Here's how the part is built. I have some questions about the finished solid (model axes, mm). Round coordinates to 2 decimals unless told otherwise and drop trailing zeros. Order: outer loops, then holes, each group sorted by start corner. A loop starts at its lowest first (then second) coordinate and runs counter-clockwise, first axis right, second up.
```python
from build123d import *

# Parameters (mm, degrees)
SKETCH1_W           = 202
SKETCH1_H           = 152
SKETCH1_R           = 7.5
BOSS_EXTRUDE1_DEPTH = 10
SKETCH2_R           = 25.4
SKETCH2_R_2         = 23.9
BOSS_EXTRUDE2_DEPTH = 1220


with BuildPart() as part:
    # Sketch1 → Boss-Extrude1 (new body)
    with BuildSketch(Plane.XY):
        with Locations((-101, 76)):
            Rectangle(SKETCH1_W, SKETCH1_H)
        with Locations((-185, 141)):
            Circle(SKETCH1_R, mode=Mode.SUBTRACT)
        with Locations((-185, 11)):
            Circle(SKETCH1_R, mode=Mode.SUBTRACT)
        with Locations((-38.177870513, 141)):
            Circle(SKETCH1_R, mode=Mode.SUBTRACT)
        with Locations((-38.177870513, 11)):
            Circle(SKETCH1_R, mode=Mode.SUBTRACT)
    extrude(amount=BOSS_EXTRUDE1_DEPTH)

    # Sketch2 → Boss-Extrude2 (add)
    with BuildSketch(Plane.XY.offset(10)):
        with Locations((-101, 76)):
            Circle(SKETCH2_R)
        with Locations((-101, 76)):
            Circle(SKETCH2_R_2, mode=Mode.SUBTRACT)
    extrude(amount=BOSS_EXTRUDE2_DEPTH)


solid = part.part
```
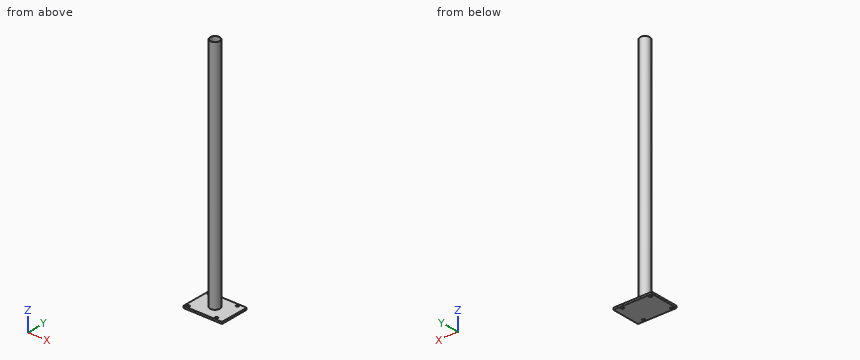
1. If we section it at A-A, the plane y = 76: Write out the boundary of the cut face in (x, z).
Evaluation:
outline: (-202, 0) - (0, 0) - (0, 10) - (-75.6, 10) - (-75.6, 1230) - (-77.1, 1230) - (-77.1, 10) - (-124.9, 10) - (-124.9, 1230) - (-126.4, 1230) - (-126.4, 10) - (-202, 10) - close
2. If we section it at C-C, the plane z = 625: Write out the boundary of the cut face in (x, y).
Evaluation:
outline: circle Ø50.8 at (-101, 76); hole circle Ø47.8 at (-101, 76)
3. I need wall thicknesses on probe 1 along Y at (x, z) = (-185, 6.75); probe 2 along X at (y, z) = (73, 988.5); probe 3 along Y at (x, z) = (-101, 818). Which ranges of each line are inside material? Lowest first, please.
Evaluation:
probe 1: y = 0 to 3.5, 18.5 to 133.5, 148.5 to 152
probe 2: x = -126.22 to -124.71, -77.29 to -75.78
probe 3: y = 50.6 to 52.1, 99.9 to 101.4
4. If we section it at B-B, the plane x = -101: Write out the boundary of the cut face in (y, z).
Evaluation:
outline: (0, 0) - (152, 0) - (152, 10) - (101.4, 10) - (101.4, 1230) - (99.9, 1230) - (99.9, 10) - (52.1, 10) - (52.1, 1230) - (50.6, 1230) - (50.6, 10) - (0, 10) - close
5. I'm going to push flat-ended pins straight in: P1, Ø3, axis at x = -115, z = 745.5, coming from the -Y side; P2, Ø9, axis at x = -185, y = 11, coming from the -Z side; P3, Ø6, axis at x = -172.5, y = 107.5, coming from the +Z side; P4, Ø6, axis at y = 76, z = 374.5, coming from the -X side. Where does each tip first touch, or does it pass through?
Evaluation:
P1: stops at y = 53.89
P2: passes through
P3: stops at z = 10
P4: stops at x = -126.4
6. If we section it at D-D, the plane x = -14: Write out the boundary of the cut face in (y, z).
Evaluation:
outline: (0, 0) - (152, 0) - (152, 10) - (0, 10) - close
